from build123d import *

# Parameters (mm, degrees)
F0_W           = 133
F0_H           = 197
F0_W_2         = 83.25
F0_H_2         = 159.5
F0_W_3         = 5
F0_H_3         = 117
F0_W_4         = 22.5
F0_H_4         = 22.5
F1_DEPTH       = 3
F2_DEPTH       = 12.5
F3_R           = 3.25
F4_DEPTH       = 2.5
F5_DEPTH       = 5
F6_R           = 10
F7_DEPTH       = 1
F16_W          = 7.5
F16_H          = 25
F17_DEPTH      = 7.5
F18_R          = 2.625
F19_DEPTH      = 162.501
F19_DEPTH_BACK = 10
F16_W_2        = 4
F16_H_2        = 36
F20_DEPTH      = 4


with BuildPart() as f1:
    # F0 (on Top) → F1 (new body)
    with BuildSketch(Plane.XY):
        with Locations((-11.25, -8.4886514246)):
            Rectangle(F0_W, F0_H)
        with Locations((-11.25, -14.7386514246)):
            Rectangle(F0_W_2, F0_H_2, mode=Mode.SUBTRACT)
        with Locations((-11.25, -14.7386514246)):
            Rectangle(F0_W_2, F0_H_2)
        with Locations((-46.25, -30.9886514246)):
            Rectangle(F0_W_3, F0_H_3, mode=Mode.SUBTRACT)
        with Locations((-36.25, -30.9886514246)):
            Rectangle(F0_W_3, F0_H_3, mode=Mode.SUBTRACT)
        with Locations((-26.25, -30.9886514246)):
            Rectangle(F0_W_3, F0_H_3, mode=Mode.SUBTRACT)
        with Locations((-16.25, -30.9886514246)):
            Rectangle(F0_W_3, F0_H_3, mode=Mode.SUBTRACT)
        with Locations((-6.25, -30.9886514246)):
            Rectangle(F0_W_3, F0_H_3, mode=Mode.SUBTRACT)
        with Locations((3.75, -30.9886514246)):
            Rectangle(F0_W_3, F0_H_3, mode=Mode.SUBTRACT)
        with Locations((13.75, -30.9886514246)):
            Rectangle(F0_W_3, F0_H_3, mode=Mode.SUBTRACT)
        with Locations((23.75, -30.9886514246)):
            Rectangle(F0_W_3, F0_H_3, mode=Mode.SUBTRACT)
        with Locations((-11.25, 43.7613485754)):
            Rectangle(F0_W_4, F0_H_4, mode=Mode.SUBTRACT)
    extrude(amount=F1_DEPTH)

    # F0 (on Top) → F2 (join)
    with BuildSketch(Plane.XY):
        with Locations((-11.25, -8.4886514246)):
            Rectangle(F0_W, F0_H)
        with Locations((-11.25, -14.7386514246)):
            Rectangle(F0_W_2, F0_H_2, mode=Mode.SUBTRACT)
    extrude(amount=F2_DEPTH)

    # F3 (on face) → F4 (cut)
    with BuildSketch(Plane.XY.offset(12.5)):
        with Locations((-65.25, -8.4886514246)):
            Circle(F3_R)
        Polygon((-77.75, 90.0113485754), (-77.75, 55.0113485754), (-52.875, 55.0113485754), (-52.875, 65.0113485754), (-10.4772727273, 65.0113485754), (10.25, 77.0113485754), (55.25, 77.0113485754), (55.25, 90.0113485754), align=None)
    extrude(amount=-F4_DEPTH, mode=Mode.SUBTRACT)

    # F3 (on face) + F4_face (on face) → F5 (join)
    with BuildSketch(Plane.XY.offset(12.5)):
        Polygon((-77.75, 90.0113485754), (-77.75, 55.0113485754), (-52.875, 55.0113485754), (-52.875, 65.0113485754), (-10.4772727273, 65.0113485754), (10.25, 77.0113485754), (55.25, 77.0113485754), (55.25, 90.0113485754), align=None)
        Polygon((-52.875, 65.0113485754), (-52.875, 55.0113485754), (-27.75, 55.0113485754), (-10.4772727273, 65.0113485754), align=None)
    with BuildSketch(Plane(origin=(-24.6626652531, 77.5848918874, 10), x_dir=(1, 0, 0), z_dir=(0, 0, 1))):
        Polygon((-53.0873347469, 12.426456688), (-53.0873347469, -22.573543312), (-28.2123347469, -22.573543312), (-28.2123347469, -12.573543312), (14.1853925258, -12.573543312), (34.9126652531, -0.573543312), (79.9126652531, -0.573543312), (79.9126652531, 12.426456688), align=None)
    extrude(amount=F5_DEPTH)

    # F6 (on face) → F7 (join)
    with BuildSketch(Plane.XY.offset(17.5)):
        with Locations((-62.75, 75.0113485754)):
            Circle(F6_R)
    extrude(amount=F7_DEPTH)

    # F9 (on offset) → F10 (revolve)
    with BuildSketch(Plane.XZ.offset(-75.0113485754)):
        with BuildLine():
            ThreePointArc((-62.75, 20.5), (-67.445725321, 19.9403364768), (-71.95, 18.5))
            Line((-71.95, 18.5), (-62.75, 18.5))
            Line((-62.75, 18.5), (-62.75, 20.5))
        make_face()
    revolve(axis=Axis((-62.75, 75.0113485754, 19.5), (0, 0, 1)))

    # F12 (on offset) → F13 (revolve)
    with BuildSketch(Plane.XZ.offset(-85.0113485754)):
        with BuildLine():
            ThreePointArc((-47.75, 19.1043560763), (-49.2352574204, 18.6687696943), (-50.25, 17.5))
            Line((-50.25, 17.5), (-47.75, 17.5))
            Line((-47.75, 17.5), (-47.75, 19.1043560763))
        make_face()
    revolve(axis=Axis((-47.75, 85.0113485754, 18.3021780381), (0, 0, 1)))

    # F12 (on offset) → F14 (revolve)
    with BuildSketch(Plane.XZ.offset(-85.0113485754)):
        with BuildLine():
            ThreePointArc((-40.25, 19.1043560763), (-41.7352574204, 18.6687696943), (-42.75, 17.5))
            Line((-42.75, 17.5), (-40.25, 17.5))
            Line((-40.25, 17.5), (-40.25, 19.1043560763))
        make_face()
    revolve(axis=Axis((-40.25, 85.0113485754, 18.3021780381), (0, 0, 1)))

    # F12 (on offset) → F15 (revolve)
    with BuildSketch(Plane.XZ.offset(-85.0113485754)):
        with BuildLine():
            ThreePointArc((-32.75, 19.1043560763), (-34.2352574204, 18.6687696943), (-35.25, 17.5))
            Line((-35.25, 17.5), (-32.75, 17.5))
            Line((-32.75, 17.5), (-32.75, 19.1043560763))
        make_face()
    revolve(axis=Axis((-32.75, 85.0113485754, 18.3021780381), (0, 0, 1)))

    # F16 (on face) → F17 (cut)
    with BuildSketch(Plane.XY.offset(12.5)):
        with Locations((51.5, 43.0113485754)):
            Rectangle(F16_W, F16_H)
        with Locations((51.5, -14.9886514246)):
            Rectangle(F16_W, F16_H)
        with Locations((51.5, -72.9886514246)):
            Rectangle(F16_W, F16_H)
    extrude(amount=-F17_DEPTH, mode=Mode.SUBTRACT)

    # F18 (on face) → F19 (cut, two sides)
    with BuildSketch(Plane.XZ.offset(-55.5113485754)) as f19_sk:
        with Locations((51.5, 8.75)):
            Circle(F18_R)
    extrude(amount=F19_DEPTH, mode=Mode.SUBTRACT)
    extrude(f19_sk.sketch, amount=-F19_DEPTH_BACK, mode=Mode.SUBTRACT)

    # F16 (on face) → F20 (cut)
    with BuildSketch(Plane.XY.offset(12.5)):
        with Locations((32.375, -3.9886514246)):
            Rectangle(F16_W_2, F16_H_2)
    extrude(amount=-F20_DEPTH, mode=Mode.SUBTRACT)


solid = f1.part
Input: part model. Units: mm. Frame: model coordinates. A direction names the side the tool comes from. Give positions to 0.01 mm unless a question says otherwise; leave off trailing zeros. Loops run counter-clockwise (first coordinate to the right, second up) from the corner with the lowest first, then second, coordinate; pieces in that order, holes last. Notation, with made-up numbers: (68, -17) - (124, -17) arc R10 ccw to (124, -2) - close; hole circle Ø10 at (-2.75, -8.5). An arc over 180 degrees is marked (long way). Use CSV: the item, a comma, the result in double quotes. Start each with the question number.
Item 1: Mould query, pull axis Z, two halves, no side actions, for faces 4 (the cylindrical face through (-68.497, -8.346, 11.268)), 5 (the flat face through (51, -15, 5)), 6 (the cylindrical face through (54.004, 60.441, 9.538)), 7 (the flat face through (-12, -7, 0)). Classes: pulls with the +Z half, pulls with the -Z half, needs draft (parallel to the pull), parting line crosses it, or undercut.
Item 2: Section A-A on x = 51.5. State how many separate pieces and enclosed holes the cut face has, then the cut area to 3 significant figures.
Item 3: Line query: line 1 (Z direction, x = 51.5, y = -100.75) (3 decimals); line 2 (Z direction, x = 51, y = -43); line 3 (X direction, y = 19, z = 8.75) (3 decimals). Output: solid intervals per line, ascending.
Item 4: Contact query for flat-ended pins moving along their axis: P1, Ø4, axis at x = 53, y = 48, coming from the +Z side; P2, Ø4, axis at x = 51.5, z = 8.75, coming from the -Y side; P3, Ø5, axis at x = -39.5, y = -56.5, coming from the +Z side. Output: stop coordinate, or through.
Item 5: Section B-B on y = 51. Return loops of the section in (x, z) (3 decimals), then the cut area to 3 significant figures.
Item 6: Reachability of faces 1 (the flat face through (-37, 60, 12.5)), 2 (the flat face through (49, -27.489, 10)), 3 (the flat face through (32, 77.011, 15)) from +Z, -Z, +X, -X, +Y, -Y: full face, straight path, thin tool, end or side. Return the list, or none.
Ans:
1,face 4,"needs draft"
1,face 5,"pulls with the +Z half"
1,face 6,"undercut"
1,face 7,"pulls with the -Z half"
2,separate pieces,"4"
2,enclosed holes,"0"
2,area,"1,450 mm2"
3,line 1,"z = 0 to 6.125, 11.375 to 12.5"
3,line 2,"z = 0 to 6.17, 11.33 to 12.5"
3,line 3,"x = -77.75 to -52.875, 30.375 to 48.875, 54.125 to 55.25"
4,P1,"stops at z = 5"
4,P2,"stops at y = 65.51"
4,P3,"stops at z = 3"
5,outline,"(-77.75, 0) - (-22.5, 0) - (-22.5, 3) - (-52.875, 3) - (-52.875, 12.5) - (-77.75, 12.5) - close; (0, 0) - (55.25, 0) - (55.25, 5) - (47.75, 5) - (47.75, 12.5) - (30.375, 12.5) - (30.375, 3) - (0, 3) - close"
5,area,"748 mm2"
6,face 1,"none"
6,face 2,"+Z, +X"
6,face 3,"+Z, +X, -Y"
